CAD build for the part. Positions are in the model's coordinates, mm. Coordinates: 2 decimals unless noted, no trailing zeros. Write each loop counter-clockwise with the first axis right and the second up, starting at its lowest first coordinate (ties: lowest second). Pieces come first, ordered by that corner, then holes. Notation, with made-up numbers: M -37,74 L -23,74 A24 ccw -23,91 Z; hole C 33,78 d10. An arc over 180 degrees is marked long. Put each result on its own line as item: value. Start each with the question number.
```python
from build123d import *

# Parameters (mm, degrees)
ESBO_O1_W                = 150
ESBO_O1_H                = 40
RESSALTO_EXTRUS_O1_DEPTH = 4
FILETE2_R                = 15
FUROS_GUIA_COM_20_0MM1_D = 20


with BuildPart() as part:
    # Esboço1 → Ressalto-extrusão1 (new, symmetric)
    with BuildSketch(Plane.XY):
        with Locations((75, 20)):
            Rectangle(ESBO_O1_W, ESBO_O1_H)
    extrude(amount=RESSALTO_EXTRUS_O1_DEPTH, both=True)

    # Filete2
    filete2_edges = [part.edges().sort_by_distance(p)[0] for p in [
        (0, 0, 0),
        (0, 40, 0),
        (150, 40, 0),
        (150, 0, 0),
    ]]
    fillet(filete2_edges, radius=FILETE2_R)

    # Furos-guia com Ø20.0mm1 (through all)
    with Locations(Plane.XY.offset(4)):
        with Locations((20, 20), (130, 20)):
            Hole(FUROS_GUIA_COM_20_0MM1_D / 2)


solid = part.part
```
(1) Slice it at B-B, the plane x = 130. Write the cut outline in (y, z).
(2) Slice it at A-A, the plane y = 22. Write the cut outline in (x, z), then the cut area to 3 significant figures.
(3) Slice it at C-C, the plane z = 2.25. Write the cut outline in (x, y).
(4) Two-plate mould, pull along Y, no slides. Class faces 1 (the face through (4.28, 4.51, 0.06)), 2 (the face through (150, 20, 0)), 3 (the face through (10.46, 23, -0.06)): +Y half, -Y half, draft (parallel to the pull), parting line (faces both ways), or undercut.
(5) Drop flat-ended pins along their axis: pin 1 (1.5 mm diameter, centred on y = 8.5, z = 1, fed in from -X); pin 2 (2 mm diameter, centred on y = 36, z = -2.5, fed in from -X). Give the stop position or say it passes through.
(6) Drill centre lines: line 1 (X direction, y = 13.5, z = 3.5); line 2 (X direction, y = 21, z = -2.5); line 3 (Y direction, x = 130, z = 0). Where is each one in solid material? Low to high. Write a range as [from, to].
(7) Slice it at D-D, the plane y = 33. Write the cut outline in (x, z).
Result set:
1. outline: M 0,-4 L 10,-4 L 10,4 L 0,4 Z; M 30,-4 L 40,-4 L 40,4 L 30,4 Z
2. outline: M 0,-4 L 10.2,-4 L 10.2,4 L 0,4 Z; M 29.8,-4 L 120.2,-4 L 120.2,4 L 29.8,4 Z; M 139.8,-4 L 150,-4 L 150,4 L 139.8,4 Z
2. area: 886 mm^2
3. outline: M 0,15 A15 ccw 15,0 L 135,0 A15 ccw 150,15 L 150,25 A15 ccw 135,40 L 15,40 A15 ccw 0,25 Z; hole C 20,20 d20; hole C 130,20 d20
4. face 1: -Y half
4. face 2: draft
4. face 3: undercut
5. pin 1: stops at x = 1.15
5. pin 2: stops at x = 3.82
6. line 1: x = [0.08, 12.4], [27.6, 122.4], [137.6, 149.92]
6. line 2: x = [0, 10.05], [29.95, 120.05], [139.95, 150]
6. line 3: y = [0, 10], [30, 40]
7. outline: M 2.31,-4 L 147.69,-4 L 147.69,4 L 2.31,4 Z
